from build123d import *

# Parameters (mm, degrees)
BASE_FLANGE1_DEPTH = 22.5
SKETCH6_R          = 1.5
CUT_EXTRUDE2_DEPTH = 47.800106837
SKETCH8_R          = 1.5
CUT_EXTRUDE3_DEPTH = 47.800106837
CUT_EXTRUDE5_START = -17.038685437
CUT_EXTRUDE5_DEPTH = 34.599471918


# Read off the part's stored shape, not the designer's step: Cut-Extrude5
# Sheet-metal steps are written as plain solids
with BuildPart() as part:
    # Sketch2 → Base-Flange1 (new, symmetric)
    with BuildSketch(Plane(origin=(0, 0, 0), x_dir=(0, 0, -1), z_dir=(1, 0, 0))):
        with BuildLine():
            Line((30, 0), (0.7366, 0))
            ThreePointArc((0.7366, 0), (0.215745145, 0.215745145), (0, 0.7366))
            Line((0, 0.7366), (0, 28))
            Line((0, 28), (-0.7366, 28))
            Line((-0.7366, 28), (-0.7366, 0.7366))
            ThreePointArc((-0.7366, 0.7366), (-0.30510971, -0.30510971), (0.7366, -0.7366))
            Line((0.7366, -0.7366), (30, -0.7366))
            Line((30, -0.7366), (30, 0))
        make_face()
    extrude(amount=BASE_FLANGE1_DEPTH, both=True)

    # Sketch6 → Cut-Extrude2 (cut, through all)
    with BuildSketch(Plane(origin=(0, 0, 0), x_dir=(-1, 0, 0), z_dir=(0, 0, -1))):
        with Locations((-20.5, 9.5)):
            Circle(SKETCH6_R)
        with Locations((20.5, 26)):
            Circle(SKETCH6_R)
    extrude(amount=-CUT_EXTRUDE2_DEPTH, mode=Mode.SUBTRACT)

    # Sketch8 → Cut-Extrude3 (cut, through all)
    with BuildSketch(Plane(origin=(0, 0, 0), x_dir=(1, 0, 0), z_dir=(0, 1, 0))):
        with Locations(Location((0, 15, 0), (0, 0, 270))):
            Circle(SKETCH8_R)
        with Locations(Location((-16, 15, 0), (0, 0, 270))):
            Circle(SKETCH8_R)
    cut_extrude3 = extrude(amount=-CUT_EXTRUDE3_DEPTH, mode=Mode.SUBTRACT)

    # Mirror1: Cut-Extrude3 across plane
    add(cut_extrude3.mirror(Plane(origin=(0, 0, 0), x_dir=(0, 0, 1), z_dir=(1, 0, 0))), mode=Mode.SUBTRACT)

    # Cut-Extrude5 outline → Cut-Extrude5 (cut)
    with BuildSketch(Plane.YZ.offset(CUT_EXTRUDE5_START)):
        with BuildLine():
            ThreePointArc((0.7366, 0.7366), (0.620934378, 0.732052343), (0.505982859, 0.718437448))
            Line((0.505982859, 0.718437448), (0.62129143, -0.009081276))
            ThreePointArc((0.62129143, -0.009081276), (0.678767189, -0.002273829), (0.7366, 0))
            Line((0.7366, 0), (26.231735093, 0))
            Line((26.231735093, 0), (26.231735093, 0.7366))
            Line((26.231735093, 0.7366), (0.7366, 0.7366))
        make_face()
    extrude(amount=CUT_EXTRUDE5_DEPTH, mode=Mode.SUBTRACT)


solid = part.part
CAD build for the part. Positions are in the model's coordinates, mm. A direction names the side the tool comes from. Give positions to 0.01 mm unless a question says otherwise; leave off trailing zeros. Write each loop counter-clockwise with the first axis right and the second up, starting at its lowest first coordinate (ties: lowest second). Pieces come first, ordered by that corner, then holes. Notation, with made-up numbers: (50.25, -30.75) -> (100.25, -30.75) arc R38 cw to (100.25, 7.25) -> close; hole circle Ø5 at (-36.75, 37.25). An arc over 180 degrees is marked (long way). Return JSON: item names as keys, results as strings.
Item 1: Band-saw the part on C-C (z = -15). List the corners of the cut face in (x, y), then the cut area to 3 significant figures.
Answer below:
{"outline": "(-22.5, -0.74) -> (-17.5, -0.74) -> (-17.5, 0) -> (-22.5, 0) -> close; (-14.5, -0.74) -> (-1.5, -0.74) -> (-1.5, 0) -> (-14.5, 0) -> close; (1.5, -0.74) -> (14.5, -0.74) -> (14.5, 0) -> (1.5, 0) -> close; (17.5, -0.74) -> (22.5, -0.74) -> (22.5, 0) -> (17.5, 0) -> close", "area": "26.5 mm2"}
Item 2: Band-saw the part on D-D (x = 16). List the corners of the cut face in (y, z), then the cut area to 3 significant figures.
Answer below:
{"outline": "(-0.74, -30) -> (0, -30) -> (0, -16.5) -> (-0.74, -16.5) -> close; (-0.74, -13.5) -> (0, -13.5) -> (0, -0.74) arc R0.74 cw to (0.62, -0.01) -> (0.51, 0.72) arc R1.47 ccw to (-0.74, -0.74) -> close; (26.23, 0) -> (28, 0) -> (28, 0.74) -> (26.23, 0.74) -> close", "area": "21.8 mm2"}
Item 3: Drop a flat-ended pin along its axis: pin 1 (14.5 mm diameter, centred on x = 5, z = -14, fed in from +Y). Give the stop position or say it passes through.
Answer below:
{"pin 1": "stops at y = 0"}
Item 4: Two-plate mould, pull along Z, no slides. Class faces 3 (the cylindrical face through (15.93, -0.36, -16.5)), 4 (the cylindrical face through (22, 9.57, 0.36)), 5 (the flat face through (-2, 27, 0.737)), 6 (the cylindrical face through (-15.93, -0.36, -16.5)): +Z half, -Z half, draft (parallel to the pull), parting line (faces both ways), or undercut.
Answer below:
{"face 3": "undercut", "face 4": "draft", "face 5": "+Z half", "face 6": "undercut"}
Item 5: Band-saw the part on A-A (x = -20.5). List the corners of the cut face in (y, z).
Answer below:
{"outline": "(-0.74, -30) -> (0, -30) -> (0, -0.74) arc R0.74 cw to (0.74, 0) -> (24.5, 0) -> (24.5, 0.74) -> (0.74, 0.74) arc R1.47 ccw to (-0.74, -0.74) -> close; (27.5, 0) -> (28, 0) -> (28, 0.74) -> (27.5, 0.74) -> close"}
Item 6: Band-saw the part on B-B (y = 14). List the corners of the cut face in (x, z).
Answer below:
{"outline": "(-22.5, 0) -> (-17.04, 0) -> (-17.04, 0.74) -> (-22.5, 0.74) -> close; (17.56, 0) -> (22.5, 0) -> (22.5, 0.74) -> (17.56, 0.74) -> close"}
Item 7: Tool access for faces 1 (the flat face through (0, 0, -12)), 2 (the flat face through (0, -0.737, -12)): list every direction of +Z, -Z, +X, -X, +Y, -Y with a clear straight run to the whole face (end or side of a thin tool).
Answer below:
{"face 1": "-Z, +X, -X, +Y", "face 2": "+Z, -Z, +X, -X, -Y"}
Item 8: Drill centre lines: probe 1 along X at (y, z) = (-0.3, -15); probe 2 along Y at (x, z) = (-8, -24); probe 3 along Z at (x, y) = (-20, 22.25). Where is each one in solid material? Low to high.
Answer below:
{"probe 1": "x = -22.5 to -17.5, -14.5 to -1.5, 1.5 to 14.5, 17.5 to 22.5", "probe 2": "y = -0.74 to 0", "probe 3": "z = 0 to 0.74"}
